Geometry: final body of the model. Coordinates: model frame, mm. A direction names the side the tool comes from. Give positions to 0.01 mm unless a question says otherwise; leave off trailing zeros. Write each loop counter-clockwise with the first axis right and the second up, starting at its lowest first coordinate (ties: lowest second). Pieces come first, ordered by that corner, then holes. Notation, with made-up numbers: M 29,-38 L 39,-38 A8 cw 39,-33 Z; hole C -30,39 d1. An arc over 180 degrees is marked long. Use one line per item in the form item = value. Start each with the question number.
Item 1: Pull-direction query (X, two-part tool) for faces 4 (the cylindrical face through (-0.358, 6.972, -19.273)), 5 (the cylindrical face through (6.5, 163.2, -12.4)), 6 (the cylindrical face through (-0.59, 2.46, -17.54)), 7 (the flat face through (-8, 152, 12)); classes: released by +X, released by -X, zero draft, split by the parting line, or undercut.
Item 2: Section query B-B on z = -22. Return loops of the section in (x, y).
Item 3: Section query C-C on y = 34. Return loops of the section in (x, z).
Item 4: Access query for faces 1 (the flat face through (0, 29, 15.5)), 2 (the cylindrical face through (-11.99, 183.13, 0.53)), 3 (the flat face through (-18, 5, 8)). Directions: +Z, -Z, +X, -X, +Y, -Y. A direction counts if a zero-diameter tool reaches every point of the face in a straight line with its end or side. Return the directions, or none.
Item 5: Material intervals for line 1 along Z through (x, y) = (0, 6); line 2 along Y through (x, z) = (8.5, 8.5); line 3 along Y through (x, z) = (-23, -5), sorted ascending. Write a range as from..to.
Item 6: Section query A-A on z = 0. Return loops of the section in (x, y).
Item 7: Contact query for flat-ended pins moving along their axis: P1, Ø4.5, axis at x = 19.05, z = 11, coming from the +Y side; P2, Ø8, axis at x = -19.05, z = 11, coming from the -Y side; P3, Ø4, axis at x = 18, z = -15.5, coming from the -Y side; P4, Ø8, axis at y = 67.5, z = -17, coming from the -X side. Output: stop coordinate, or through.
from build123d import *

# Parameters (mm, degrees)
CUT_EXTRUDE1_DEPTH = 2
CUT_EXTRUDE2_DEPTH = 1.5
SKETCH7_R          = 2.75
CUT_EXTRUDE3_DEPTH = 9
SKETCH8_R          = 4.5
CUT_EXTRUDE4_DEPTH = 5
CIRPATTERN1_COUNT  = 3
CIRPATTERN2_COUNT  = 3


with BuildPart() as part:
    # Sketch1 → Revolve1 (revolve)
    with BuildSketch(Plane.XY):
        Polygon((0, 0), (28, 0), (28, 9), (17.5, 9), (17.5, 152), (14, 152), (14, 174), (12, 174), (12, 192), (10, 192), (10, 220), (8, 220), (8, 227), (0, 227), align=None)
    revolve(axis=Axis((0, 340.077659461, 0), (0, -1, 0)))

    # Sketch2 → Cut-Extrude1 (cut)
    with BuildSketch(Plane.XY.offset(17.5)):
        with BuildLine():
            Line((3, 44), (3, 14))
            ThreePointArc((3, 14), (0, 11), (-3, 14))
            Line((-3, 14), (-3, 44))
            ThreePointArc((-3, 44), (0, 47), (3, 44))
        make_face()
    extrude(amount=-CUT_EXTRUDE1_DEPTH, mode=Mode.SUBTRACT)

    # Sketch3 → Cut-Extrude2 (cut)
    with BuildSketch(Plane.XY.offset(14)):
        with BuildLine():
            Line((2.5, 164), (2.5, 155))
            ThreePointArc((2.5, 155), (0, 152.5), (-2.5, 155))
            Line((-2.5, 155), (-2.5, 164))
            ThreePointArc((-2.5, 164), (0, 166.5), (2.5, 164))
        make_face()
    extrude(amount=-CUT_EXTRUDE2_DEPTH, mode=Mode.SUBTRACT)

    # Sketch7 → Cut-Extrude3 (cut)
    with BuildSketch(Plane.XZ):
        with Locations((0, -22)):
            Circle(SKETCH7_R)
    cut_extrude3 = extrude(amount=-CUT_EXTRUDE3_DEPTH, mode=Mode.SUBTRACT)

    # Sketch8 → Cut-Extrude4 (cut)
    with BuildSketch(Plane.XZ):
        with Locations((0, -22)):
            Circle(SKETCH8_R)
    cut_extrude4 = extrude(amount=-CUT_EXTRUDE4_DEPTH, mode=Mode.SUBTRACT)

    # CirPattern1: Cut-Extrude3 ×3 about axis
    cirpattern1_axis = Axis((0, 0, 0), (0, 1, 0))
    for i in range(1, CIRPATTERN1_COUNT):
        add(cut_extrude3.rotate(cirpattern1_axis, i * 360 / CIRPATTERN1_COUNT), mode=Mode.SUBTRACT)

    # CirPattern2: Cut-Extrude4 ×3 about axis
    cirpattern2_axis = Axis((0, 0, 0), (0, 1, 0))
    for i in range(1, CIRPATTERN2_COUNT):
        add(cut_extrude4.rotate(cirpattern2_axis, i * 360 / CIRPATTERN2_COUNT), mode=Mode.SUBTRACT)


solid = part.part
Answer sheet:
q1.face_4 = undercut
q1.face_5 = split by the parting line
q1.face_6 = undercut
q1.face_7 = zero draft
q2.outline = M -17.32,0 L -4.5,0 L -4.5,5 L -2.75,5 L -2.75,9 L -17.32,9 Z; M 2.75,5 L 4.5,5 L 4.5,0 L 17.32,0 L 17.32,9 L 2.75,9 Z
q3.outline = M -3,15.5 L -3,17.24 A17.5 ccw long 3,17.24 L 3,15.5 Z
q4.face_1 = +Z
q4.face_2 = +Y
q4.face_3 = -Y
q5.line_1 = -28..-24.75, -19.25..28
q5.line_2 = 0..174
q5.line_3 = 0..9
q6.outline = M -28,0 L 28,0 L 28,9 L 17.5,9 L 17.5,152 L 14,152 L 14,174 L 12,174 L 12,192 L 10,192 L 10,220 L 8,220 L 8,227 L -8,227 L -8,220 L -10,220 L -10,192 L -12,192 L -12,174 L -14,174 L -14,152 L -17.5,152 L -17.5,9 L -28,9 Z
q7.P1 = through
q7.P2 = 5
q7.P3 = 0
q7.P4 = -11.72
